Autodesk Inventor part; units mm, degrees
ref_plane "YZ Plane" through (0, 0, 0) normal (1, 0, 0) x (0, 1, 0)
ref_plane "XZ Plane" through (0, 0, 0) normal (0, 1, 0) x (-1, 0, 0)
ref_plane "XY Plane" through (0, 0, 0) normal (0, 0, 1) x (1, 0, 0)
sketch "Sketch1" plane through (0, 0, 0) normal (0, 1, 0) x (-1, 0, 0)
  circle A0 centre (0, 0) radius 8
  dimension "d0" = 16
extrude "Extrusion1" add sketch "Sketch1" against normal blind 5
sketch "Sketch2" plane through (0, 0, 0) normal (0, 1, 0) x (1, 0, 0)
  circle A0 centre (0, 0) radius 12
  dimension "d3" = 24
extrude "Extrusion2" add sketch "Sketch2" along normal blind 16
sketch "Sketch3" plane through (0, 16, 0) normal (0, 1, 0) x (1, 0, 0)
  circle A0 centre (0, 0) radius 12
  circle A1 centre (0, 0) radius 13.5
  dimension "d6" = 1.5
extrude "Extrusion3" add sketch "Sketch3" along normal blind 6 contours A0 | A1
sketch "Sketch4" plane through (0, 22, 0) normal (0, 1, 0) x (1, 0, 0)
  circle A0 centre (0, 0) radius 7
  dimension "d9" = 14
extrude "Extrusion4" add sketch "Sketch4" along normal blind 9
sketch "Sketch5" plane through (0, 22, 0) normal (0, 1, 0) x (1, 0, 0)
  circle A0 centre (0, 0) radius 13.5
extrude "Extrusion5" add sketch "Sketch5" along normal blind 6.75 draft -55
properties part number "OXYGEN SENSOR"
For this review, take the finished solid that the model builds, in its own axes (mm). A direction names the side the tool comes from. Give positions to 0.01 mm unless a question says otherwise; leave off trailing zeros. Write each loop counter-clockwise with the first axis right and the second up, starting at its lowest first coordinate (ties: lowest second). Pieces come first, ordered by that corner, then holes. Notation, with made-up numbers: M 5,48 L 20,48 A19 ccw 20,57 Z; hole C 20,10 d2. An arc over 180 degrees is marked long. Answer as a JSON object with one key per item and string values. Group by question number.
Item 1: Consider section C-C on y = 17.5. Write out the cut boundary in (x, z).
Item 2: Consider section B-B on x = 0. Write out the cut boundary in (y, z).
Item 3: Tool access review of faces 1 (the flat face through (-12, 16, 2)), 2 (the cylindrical face through (-2.93, 18.96, -13.18)), 3 (the cylindrical face through (6.466, 28.745, -2.681)): name each direction out of +Z, -Z, +X, -X, +Y, -Y from which nothing blocks a thin tool from reaching the whole face with its end or side.
Item 4: For pin 1 Ø5 at (x, y) = (1, 12) entering from -Z; pin 2 Ø1.5 at (x, z) = (8.5, 3.5) entering from +Y; pin 3 Ø3 at (x, y) = (-8, 23) entering from +Z, all flat-tipped, find the tip position at first contact; note any pin that passes through.
Item 5: Consider section A-A on z = 0. Write out the cut boundary in (x, y).
Item 6: Consider section D-D on y = 22.5. Write out the cut boundary in (x, z).
Item 7: For probe 1 along Z at (x, y) = (-0.25, 4); probe 2 along Z at (x, y) = (-11, 20.5); probe 3 along Y at (x, z) = (3, -11), list the stretches that pass through material, from the lowest coordinate up. Write a range as [from, to].
Check result:
{
 "1": {"outline": "C 0,0 d27"},
 "2": {"outline": "M -5,-8 L 0,-8 L 0,-12 L 16,-12 L 16,-13.5 L 22,-13.5 L 26.55,-7 L 31,-7 L 31,7 L 26.55,7 L 22,13.5 L 16,13.5 L 16,12 L 0,12 L 0,8 L -5,8 Z"},
 "3": {"face 1": "-Y", "face 2": "+Y, -Y", "face 3": "+Y"},
 "4": {"pin 1": "stops at z = -12", "pin 2": "stops at y = 25.54", "pin 3": "stops at z = 11.61"},
 "5": {"outline": "M -13.5,16 L -12,16 L -12,0 L -8,0 L -8,-5 L 8,-5 L 8,0 L 12,0 L 12,16 L 13.5,16 L 13.5,22 L 7,26.55 L 7,31 L -7,31 L -7,26.55 L -13.5,22 Z"},
 "6": {"outline": "C 0,0 d25.57"},
 "7": {"probe 1": "z = [-12, 12]", "probe 2": "z = [-7.83, 7.83]", "probe 3": "y = [0, 23.47]"}
}
